The drawing under review shows one solid part. Ordinate dimensions are in mm from its lowest x, y, z. A direction names the side the tool comes from. Give positions to 0.01 mm unless a question says otherwise; leave off trailing zeros. Loops run counter-clockwise (first coordinate to the right, second up) from the corner with the lowest first, then second, coordinate; pieces in that order, holes last. Notation, with made-up numbers: M 9,57.5 L 38,57.5 A30 cw 38,93.5 Z; hole C -23.75,69.25 d9. An arc over 180 degrees is marked long. Put each result on its own line as item: value. Start each with the question number.
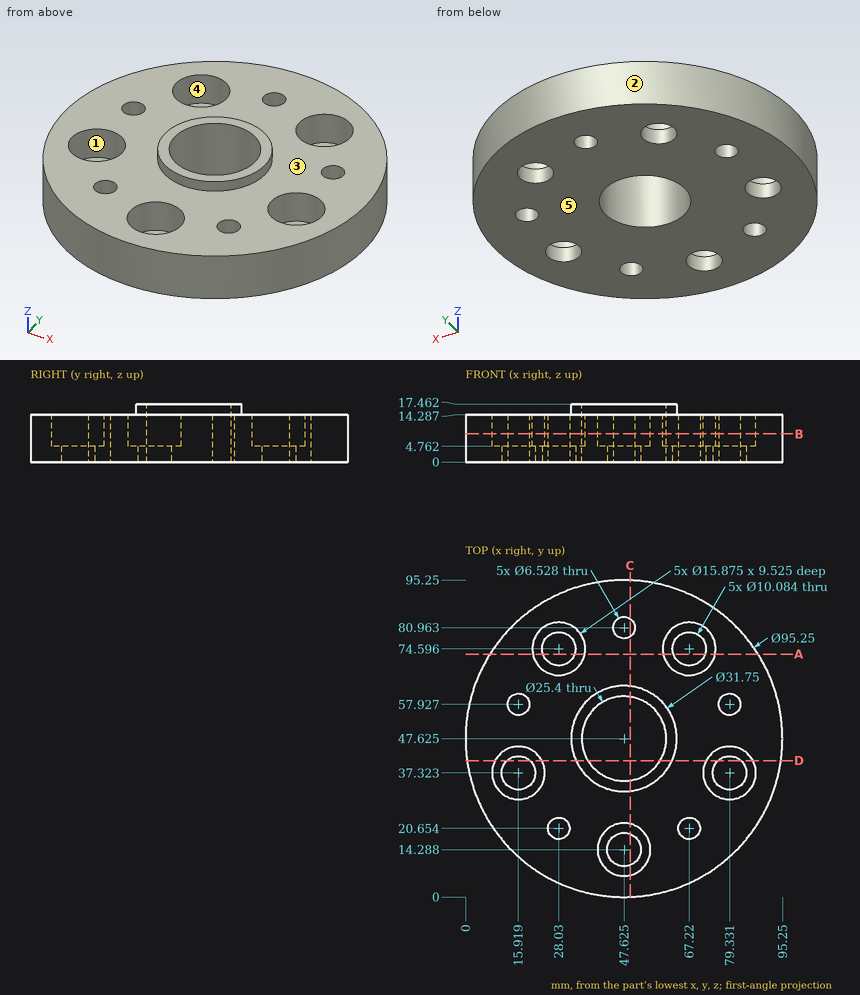
Item 1: Draft analysis for pull direction Y (two halves, no side actions). For the marked faces 1, 2 and 3, state which applies: +Y half, -Y half, draft (parallel to the pull), parting line (faces both ways), or undercut.
Item 2: Consider section B-B, the plane z = 8.5. Give the number of separate pieces and of enclosed holes in the cut face, plus the area to 3 significant figures.
Item 3: Clearance check with flat-ended pins moving along their axes: pin 1 Ø10 at (y, z) = (31.5, 12) entering from +X; pin 2 Ø5 at (x, y) = (62.5, 23.5) entering from +Z; pin 3 Ø5 at (x, y) = (80.5, 40) entering from +Z; pin 4 Ø5 at (x, y) = (61.5, 42.5) entering from -Z. State where each tip first meets the part, or that it passes through.
Item 4: Consider section D-D, the plane y = 41. Write out the cut boundary in (x, z) (1 decimal).
Item 5: To check wall thickness, follow L1, parallel to Y at x = 72, z = 12 (1 decimal); L2, parallel to X at y = 20.5, z = 2.75; L3, parallel to Y at x = 79, z = 12 (1 decimal). State the ranges of each line that lie inside material, in increasing order. Write a range as [from, to].
Item 6: Tool access review of the marked faces 4 and 5: name each direction out of +Z, -Z, +X, -X, +Y, -Y from which nothing blocks a thin tool from reaching the whole face with its end or side.
Item 7: Consider section A-A, the plane y = 73. Write out the cut boundary in (x, z) (1 decimal).
Item 8: Consider section C-C, the plane x = 49.5. Write out the cut boundary in (y, z) (1 decimal).
Report:
1. face 1: undercut
1. face 2: parting line
1. face 3: draft
2. separate pieces: 1
2. enclosed holes: 11
2. area: 5,460 mm²
3. pin 1: x = 93.93
3. pin 2: z = 14.29
3. pin 3: z = 4.76
3. pin 4: z = 0
4. outline: M 0.5,0 L 12.5,0 L 12.5,4.8 L 8.9,4.8 L 8.9,14.3 L 0.5,14.3 Z; M 19.4,0 L 36.8,0 L 36.8,17.5 L 33.2,17.5 L 33.2,14.3 L 23,14.3 L 23,4.8 L 19.4,4.8 Z; M 58.5,0 L 75.9,0 L 75.9,4.8 L 72.3,4.8 L 72.3,14.3 L 62.1,14.3 L 62.1,17.5 L 58.5,17.5 Z; M 82.8,0 L 94.8,0 L 94.8,14.3 L 86.4,14.3 L 86.4,4.8 L 82.8,4.8 Z
5. L1: [6.7, 34.3], [40.4, 68.3], [80.9, 88.5]
5. L2: [8.48, 24.77], [31.29, 63.96], [70.48, 86.77]
5. L3: [11.8, 29.4], [45.3, 54.7], [61.2, 83.5]
6. face 4: +Z
6. face 5: -Z, +X, -X, +Y, -Y
7. outline: M 7.3,0 L 23.2,0 L 23.2,4.8 L 20.3,4.8 L 20.3,14.3 L 7.3,14.3 Z; M 32.8,0 L 62.4,0 L 62.4,4.8 L 59.4,4.8 L 59.4,14.3 L 35.8,14.3 L 35.8,4.8 L 32.8,4.8 Z; M 72,0 L 87.9,0 L 87.9,14.3 L 75,14.3 L 75,4.8 L 72,4.8 Z
8. outline: M 0,0 L 9.6,0 L 9.6,4.8 L 6.6,4.8 L 6.6,14.3 L 0,14.3 Z; M 19,0 L 35.1,0 L 35.1,17.5 L 31.9,17.5 L 31.9,14.3 L 22,14.3 L 22,4.8 L 19,4.8 Z; M 60.2,0 L 78.3,0 L 78.3,14.3 L 63.4,14.3 L 63.4,17.5 L 60.2,17.5 Z; M 83.6,0 L 95.2,0 L 95.2,14.3 L 83.6,14.3 Z
